Part model, mm, in its own coordinate system. A direction names the side the tool comes from. Coordinates: 2 decimals unless noted, no trailing zeros. Order: outer loops, then holes, each group sorted by start corner. A loop starts at its lowest first (then second) coordinate and runs counter-clockwise, first axis right, second up.
1) Cut at B-B (y = 0). List the corners of the cut face in (x, z).
2) Wall check: L1, parallel to Y at x = -7, z = 0.75; L2, parallel to X at y = 28, z = 0.25; L3, parallel to Y at x = 3.75, z = 3.75. Give the ranges that are in metal, low to high.
3) Cut at C-C (y = 16). List the corners of the cut face in (x, z), and give its area (3 significant figures).
4) Pin check, flat tips, straight feed: pin 1 Ø4.5 at (x, z) = (-3, -3) entering from -Y; pin 2 Ø4 at (y, z) = (13, -6) entering from +X; pin 3 Ø8 at (y, z) = (15.5, -4.5) entering from +X; pin 4 Ø1 at (x, y) = (-2, -1.5) entering from -Z. Stop position of each tip, or through.
5) Cut at A-A (y = -7). List the corners of the cut face in (x, z).
6) Mould opens along Z. For faces 1 (the cylindrical face through (7.63, -0.14, -2.4)), 2 (the flat face through (-1.6, 10, 3.3)), 3 (the cylindrical face through (-0.11, 0.05, -2.25)), 4 (the flat face through (-2, -2.25, 2)) say: +Z half, -Z half, draft (parallel to the pull), parting line (faces both ways), or undercut.
7) Tool access for faces 5 (the flat face through (-2, 2.25, 2)), 6 (the flat face through (0, -14.5, 0)), 7 (the cylindrical face through (-3, 20, 0)), 8 (the flat face through (1.6, -10, 3.3)): list every direction of +Z, -Z, +X, -X, +Y, -Y with a clear straight run to the whole face (end or side of a thin tool).
```python
from build123d import *

# Parameters (mm, degrees)
ESBO_O2_R                  = 2.25
CORTE_EXTRUS_O2_DEPTH      = 17
ESBO_O7_R                  = 2.25
CORTE_EXTRUS_O6_DEPTH      = 3.070552483
CORTE_EXTRUS_O6_DEPTH_BACK = 18.525365704
CUT_EXTRUDE1_DEPTH         = 2.25
FILLET1_R                  = 0.5
CHAMFER1_SIZE              = 0.25
CHAMFER4_SIZE              = 0.25


with BuildPart() as part:
    # Esboço1 → Revolução1 (revolve)
    with BuildSketch(Plane.XY):
        Polygon((0, 30), (3, 30), (3, 10), (8, 10), (8, -10), (3, -10), (3, -14.5), (0, -14.5), (0, 0), align=None)
    revolve(axis=Axis((0, 0, 0), (0, 1, 0)))

    # Esboço2 → Corte-extrusão2 (cut, through all)
    with BuildSketch(Plane.ZY.offset(8)):
        Circle(ESBO_O2_R)
    extrude(amount=-CORTE_EXTRUS_O2_DEPTH, mode=Mode.SUBTRACT)

    # Esboço7 → Corte-extrusão6 (cut, two sides)
    with BuildSketch(Plane(origin=(-6.92820323, 0, 4), x_dir=(0.258819045, 0, 0.965925826), z_dir=(-0.965925826, 0, 0.258819045))) as corte_extrus_o6_sk:
        Circle(ESBO_O7_R)
    extrude(amount=CORTE_EXTRUS_O6_DEPTH, mode=Mode.SUBTRACT)
    extrude(corte_extrus_o6_sk.sketch, amount=-CORTE_EXTRUS_O6_DEPTH_BACK, mode=Mode.SUBTRACT)

    # Sketch1 → Cut-Extrude1 (cut, symmetric)
    with BuildSketch(Plane(origin=(0, 0, 0), x_dir=(1, 0, 0), z_dir=(0, 1, 0))):
        Polygon((8, 0), (-10.844388007, 0), (-10.495748768, -4.955920946), align=None)
    extrude(amount=CUT_EXTRUDE1_DEPTH, both=True, mode=Mode.SUBTRACT)

    # Fillet1
    fillet1_edges = [part.edges().sort_by_distance(p)[0] for p in [
        (-3, -10, 0),
        (-3, 10, 0),
    ]]
    fillet(fillet1_edges, radius=FILLET1_R)

    # Chamfer1
    chamfer1_edges = [part.edges().sort_by_distance(p)[0] for p in [
        (-3, -14.5, 0),
        (-3, 30, 0),
    ]]
    chamfer(chamfer1_edges, length=CHAMFER1_SIZE)

    # Chamfer4
    chamfer4_edges = [part.edges().sort_by_distance(p)[0] for p in [
        (-8, -10, 0),
        (-8, 10, 0),
    ]]
    chamfer(chamfer4_edges, length=CHAMFER4_SIZE)


solid = part.part
```
Geometry check:
1. outline: (-7.68, -2.25) arc R8 ccw to (7.68, -2.25) - close; (-5.39, 5.92) - (7.62, 2.43) arc R8 ccw to start
2. L1: y = -10 to -2.25, 2.25 to 10
2. L2: x = -2.99 to 2.99
2. L3: y = -10 to 10
3. outline: circle Ø6 at (0, 0)
3. area: 28.3 mm2
4. pin 1: stops at y = -14.5
4. pin 2: passes through
4. pin 3: stops at x = 2.96
4. pin 4: stops at z = -7.86
5. outline: circle Ø16 at (0, 0)
6. face 1: parting line
6. face 2: draft
6. face 3: undercut
6. face 4: undercut
7. face 5: -X
7. face 6: +Z, -Z, +X, -X, -Y
7. face 7: +Y
7. face 8: -Y
